Check sheet for the modelled part. Datum: model origin and axes. Units: mm. Give positions to 0.01 mm unless a question says otherwise; leave off trailing zeros. Loops run counter-clockwise (first coordinate to the right, second up) from the corner with the lowest first, then second, coordinate; pieces in that order, holes last. Notation, with made-up numbers: (-16, 42.5) - (-3, 42.5) arc R4 ccw to (-3, 47.5) - close; hole circle Ø7 at (20.25, -23.75). An arc over 180 degrees is marked (long way). Answer in a Markdown table with one row per item. Add a question column.
(1) Go/stop test with flat-tipped pins: P1, Ø10, axis at x = 15, y = -25, coming from the -Z side; P2, Ø5, axis at x = -10, y = -38, coming from the +Z side; P3, Ø7.5, axis at x = 0, z = 53.848, coming from the -Y side; P4, Ø14.5, axis at x = 53.848, z = 0, coming from the -Y side. Record where each tip stops, or that it passes through.
(2) Sectioned sample at B-B on x = 0. Enter the section's corners in (y, z), then the cut area to 3 significant figures.
(3) Sectioned sample at D-D on y = -3. Enter the section's corners in (x, z), then the cut area to 3 significant figures.
(4) Thickness scan on L1, parallel to X at y = -6, z = 0; L2, parallel to Z at x = 0, y = -33; L3, parallel to X at y = -11.5, z = 5. Record the ranges inside material, lowest first.
(5) Sectioned sample at A-A on z = 0. Enter the section's corners in (x, y), then the cut area to 3 significant figures.
(6) Sectioned sample at C-C on y = -40. Enter the section's corners in (x, z), then the cut area to 3 significant figures.
(7) Draft check along X on faces 1 (the face through (-0.827, -9.392, 60.144)), 2 (the face through (21.633, -36.65, -28.214)), 3 (the face through (18, -19.05, 37)). Enter one of: released by +X, released by -X, zero draft, split by the parting line, or undercut.
from build123d import *

# Parameters (mm, degrees)
F2_R     = 3.048
F3_R     = 6.35
F4_DEPTH = 53.849


with BuildPart() as f1:
    # F0 (on Right) → F1 (revolve)
    with BuildSketch(Plane.YZ):
        Polygon((-53.848, 19.05), (0, 19.05), (0, 89.154), (-19.05, 89.154), (-19.05, 35.553055), (-53.848, 35.553055), align=None)
    revolve(axis=Axis((0, -0.230861, 0), (0, -1, 0)))

    # F2
    f2_edges = [f1.edges().sort_by_distance(p)[0] for p in [
        (0, -19.05, -89.154),
        (0, -19.05, -35.553055),
        (0, -53.848, -35.553055),
    ]]
    fillet(f2_edges, radius=F2_R)

    # F3 (on Front) → F4 (cut, through all)
    with BuildSketch(Plane.XZ):
        with Locations((0, 53.848)):
            Circle(F3_R)
        with Locations((53.848, 0)):
            Circle(F3_R)
        with Locations((-53.848, 0)):
            Circle(F3_R)
        with Locations((0, -53.848)):
            Circle(F3_R)
    extrude(amount=F4_DEPTH, mode=Mode.SUBTRACT)


solid = f1.part
Reply:
| question | item | result |
|---|---|---|
| 1 | P1 | z = -34.12 |
| 1 | P2 | z = 34.75 |
| 1 | P3 | through |
| 1 | P4 | y = -19.05 |
| 2 | outline | (-53.85, -32.51) arc R3.05 ccw to (-50.8, -35.55) - (-22.1, -35.55) arc R3.05 cw to (-19.05, -38.6) - (-19.05, -47.5) - (0, -47.5) - (0, -19.05) - (-53.85, -19.05) - close; (-53.85, 19.05) - (0, 19.05) - (0, 47.5) - (-19.05, 47.5) - (-19.05, 38.6) arc R3.05 cw to (-22.1, 35.55) - (-50.8, 35.55) arc R3.05 ccw to (-53.85, 32.51) - close; (-19.05, -86.11) arc R3.05 ccw to (-16, -89.15) - (0, -89.15) - (0, -60.2) - (-19.05, -60.2) - close; (-19.05, 60.2) - (0, 60.2) - (0, 89.15) - (-16, 89.15) arc R3.05 ccw to (-19.05, 86.11) - close |
| 2 | area | 3,330 mm^2 |
| 3 | outline | circle Ø178.31 at (0, 0); hole circle Ø12.7 at (-53.85, 0); hole circle Ø38.1 at (0, 0); hole circle Ø12.7 at (0, -53.85); hole circle Ø12.7 at (0, 53.85); hole circle Ø12.7 at (53.85, 0) |
| 3 | area | 23,300 mm^2 |
| 4 | L1 | -89.15 to -60.2, -47.5 to -19.05, 19.05 to 47.5, 60.2 to 89.15 |
| 4 | L2 | -35.55 to -19.05, 19.05 to 35.55 |
| 4 | L3 | -89.01 to -57.76, -49.93 to -18.38, 18.38 to 49.93, 57.76 to 89.01 |
| 5 | outline | (-89.15, -16) arc R3.05 ccw to (-86.11, -19.05) - (-60.2, -19.05) - (-60.2, 0) - (-89.15, 0) - close; (-47.5, -19.05) - (-38.6, -19.05) arc R3.05 cw to (-35.55, -22.1) - (-35.55, -50.8) arc R3.05 ccw to (-32.51, -53.85) - (-19.05, -53.85) - (-19.05, 0) - (-47.5, 0) - close; (19.05, -53.85) - (32.51, -53.85) arc R3.05 ccw to (35.55, -50.8) - (35.55, -22.1) arc R3.05 cw to (38.6, -19.05) - (47.5, -19.05) - (47.5, 0) - (19.05, 0) - close; (60.2, -19.05) - (86.11, -19.05) arc R3.05 ccw to (89.15, -16) - (89.15, 0) - (60.2, 0) - close |
| 5 | area | 3,330 mm^2 |
| 6 | outline | circle Ø71.11 at (0, 0); hole circle Ø38.1 at (0, 0) |
| 6 | area | 2,830 mm^2 |
| 7 | face 1 | undercut |
| 7 | face 2 | split by the parting line |
| 7 | face 3 | zero draft |
